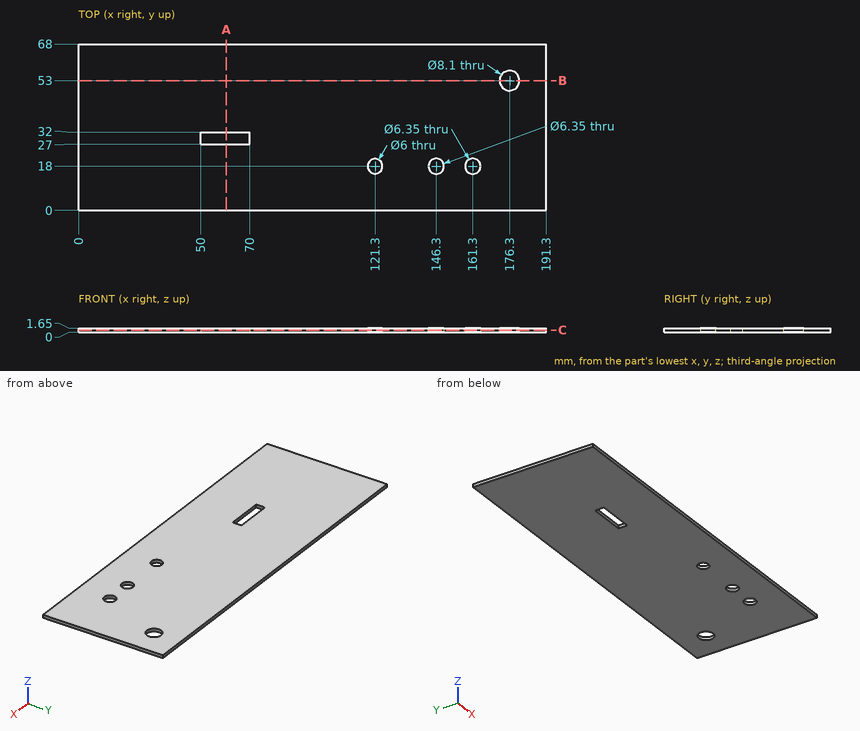
For this review, use the dimensioned drawing (mm, ordinates from the lowest corner) and the shaded views. Give positions to 0.01 mm unless a question says otherwise; leave off trailing zeros. Order: outer loops, then holes, each group sorted by start corner. A loop starts at its lowest first (then second) coordinate and runs counter-clockwise, first axis right, second up. Notation, with made-up numbers: M -36,84 L 3,84 A29 ccw 3,115 Z; hole C 65,59 d2. An arc over 180 degrees is marked long. One line per question, with ' | ' between items. Start each with the question number.
1) Consider section A-A, the plane x = 60.5. Give the boundary of the cut face in (y, z), then the cut area to 3 significant figures.
2) Clearance check with a flat-ended pin moving along its axis: P1, Ø5, axis at x = 146.3, y = 18, coming from the +Z side. State where the tip first meets the part, or that it passes through.
3) Consider section C-C, the plane z = 0.9. Give the boundary of the cut face in (x, y) (3 decimals), then the cut area to 3 significant figures.
4) Consider section B-B, the plane y = 53. Give the boundary of the cut face in (x, z), then the cut area to 3 significant figures.
5) Wall thickness on L1, parallel to Y at x = 176.3, z = 1.3; L2, parallel to Y at x = 161.3, z = 1.1 (3 decimals): over which ranges is each line inside the solid? List them lowest first. Write a range as from..to.
Found:
1) outline: M 0,0 L 27,0 L 27,1.65 L 0,1.65 Z; M 32,0 L 68,0 L 68,1.65 L 32,1.65 Z | area: 104 mm²
2) P1: passes through
3) outline: M 0,0 L 191.3,0 L 191.3,68 L 0,68 Z; hole M 50,27 L 70,27 L 70,32 L 50,32 Z; hole C 121.3,18 d6; hole C 146.3,18 d6.35; hole C 161.3,18 d6.35; hole C 176.3,53 d8.1 | area: 12,800 mm²
4) outline: M 0,0 L 172.25,0 L 172.25,1.65 L 0,1.65 Z; M 180.35,0 L 191.3,0 L 191.3,1.65 L 180.35,1.65 Z | area: 302 mm²
5) L1: y = 0..48.95, 57.05..68 | L2: y = 0..14.825, 21.175..68
